```python
from build123d import *

# Parameters (mm, degrees)
SKETCH1_R           = 32.5
BOSS_EXTRUDE1_DEPTH = 219.233663
SKETCH2_R           = 26.832853827
CUT_EXTRUDE1_DEPTH  = 224.999774536
CHAMFER1_SIZE       = 5.867198
CHAMFER1_SIZE_2     = 3.387428


with BuildPart() as part:
    # Sketch1 → Boss-Extrude1 (new body)
    with BuildSketch(Plane(origin=(0, 0, 0), x_dir=(1, 0, 0), z_dir=(0, 1, 0))):
        with Locations(Location((0, 0, 0), (0, 0, 90))):
            Circle(SKETCH1_R)
    extrude(amount=BOSS_EXTRUDE1_DEPTH)

    # Sketch2 → Cut-Extrude1 (cut, through all)
    with BuildSketch(Plane(origin=(0, 0, 0), x_dir=(1, 0, 0), z_dir=(0, 1, 0))):
        with Locations(Location((0, 0, 0), (0, 0, 90))):
            Circle(SKETCH2_R)
    extrude(amount=CUT_EXTRUDE1_DEPTH, mode=Mode.SUBTRACT)

    # Chamfer1
    # the kernel refuses this chamfer: 5.867198, 3.387428 mm, written as the material it takes off along each edge
    with BuildSketch(Plane(origin=(0, 219.233663, 0), x_dir=(0, 0, -1), z_dir=(1, 0, 0))) as chamfer1_piece_1:
        Polygon((32.5, -CHAMFER1_SIZE), (32.5 - CHAMFER1_SIZE_2, 0), (32.5, 0), align=None)
    revolve(axis=Axis((0, 219.233663, 0), (0, 1, 0)), mode=Mode.SUBTRACT)
    with BuildSketch(Plane(origin=(0, 0, 0), x_dir=(0, 0, -1), z_dir=(1, 0, 0))) as chamfer1_piece_2:
        Polygon((32.5, CHAMFER1_SIZE_2), (32.5 - CHAMFER1_SIZE, 0), (32.5, 0), align=None)
    revolve(axis=Axis((0, 0, 0), (0, 1, 0)), mode=Mode.SUBTRACT)


solid = part.part
```
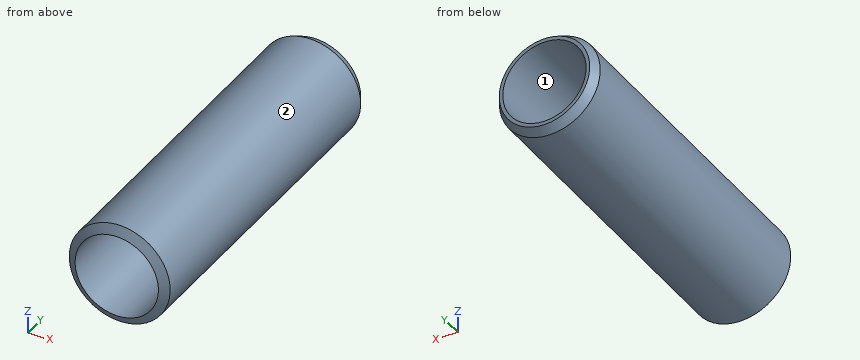
Model file for the job. Use its own axes, mm. Face numbers are marked on the shaded views. Give positions to 0.01 mm unless a question says otherwise; leave off trailing zeros. Write each loop counter-clockwise with the first axis right and the second up, starting at its lowest first coordinate (ties: lowest second). Pieces come first, ordered by that corner, then holes. Notation, with made-up numbers: (82.25, 10) - (93.25, 10) arc R10 cw to (93.25, 20) - close; hole circle Ø8 at (-27.75, -15.75). An arc over 180 degrees is marked (long way). One line per question, with ' | ' between items. Start each with the question number.
(1) Pin check, flat tips, straight feed: P1, Ø1, axis at x = 25, y = 83, coming from the +Z side; P2, Ø8, axis at x = -17.5, y = 92, coming from the +Z side; P3, Ø4, axis at y = 141, z = -7.5, coming from the -X side. Stop position of each tip, or through.
(2) Slice it at C-C on y = 189. Write the cut outline in (x, z), plus the area to 3 significant figures.
(3) Slice it at B-B on x = 0. Write the cut outline in (y, z), plus the area to 3 significant figures.
(4) Slice it at A-A on z = 0. Write the cut outline in (x, y), plus the area to 3 significant figures.
(5) Wall check: line 1 along X through (y, z) = (98.5, 0); line 2 along Z through (x, y) = (-1, 141); line 3 along Z through (x, y) = (4, 42). Give the ranges that are in metal, low to high. Write a range as from..to.
(6) Two-plate mould, pull along X, no slides. Class the marked faces 1 and 2: +X half, -X half, draft (parallel to the pull), parting line (faces both ways), or undercut.
Results below:
1) P1: z = 21.35 | P2: z = 29.56 | P3: x = -32.03
2) outline: circle Ø65 at (0, 0); hole circle Ø53.67 at (0, 0) | area: 1,060 mm^2
3) outline: (0.12, -26.83) - (3.39, -32.5) - (213.37, -32.5) - (219.23, -29.11) - (219.23, -26.83) - close; (0.12, 26.83) - (219.23, 26.83) - (219.23, 29.11) - (213.37, 32.5) - (3.39, 32.5) - close | area: 2,450 mm^2
4) outline: (-32.5, 3.39) - (-26.83, 0.12) - (-26.83, 219.23) - (-29.11, 219.23) - (-32.5, 213.37) - close; (26.83, 0.12) - (32.5, 3.39) - (32.5, 213.37) - (29.11, 219.23) - (26.83, 219.23) - close | area: 2,450 mm^2
5) line 1: -32.5..-26.83, 26.83..32.5 | line 2: -32.48..-26.81, 26.81..32.48 | line 3: -32.25..-26.53, 26.53..32.25
6) face 1: undercut | face 2: parting line
